Could you check a few things on this model? Use its own coordinates, in mm. A direction names the side the tool comes from. Give positions to 0.01 mm unless a question says otherwise; leave off trailing zeros. Order: outer loops, then holes, each group sorted by start corner. A loop starts at its lowest first (then second) coordinate and runs counter-clockwise, first axis right, second up. Notation, with made-up numbers: (-23, 88) -> (-1, 88) arc R24 ccw to (-1, 113) -> close; hole circle Ø11 at (68.5, 32). An arc over 180 degrees is marked (long way). Write each question's results on one line, items separated by ' | '.
```python
from build123d import *

# Parameters (mm, degrees)
F0_W     = 101.6
F0_H     = 76.2
F1_DEPTH = 76.2
F3_DEPTH = 76.201
F2_W     = 63.5
F2_H     = 25.4
F4_DEPTH = 63.5
F2_W_2   = 12.7
F2_H_2   = 31.75
F5_DEPTH = 50.8
F6_R     = 5.08
F7_R     = 5.08


with BuildPart() as f1:
    # F0 (on Front) → F1 (new body)
    with BuildSketch(Plane.XZ):
        Rectangle(F0_W, F0_H)
    extrude(amount=F1_DEPTH)

    # F2 (on face) → F3 (cut, through all)
    with BuildSketch(Plane.XZ.offset(76.2)):
        with BuildLine():
            ThreePointArc((-25.4, 38.1), (0, 12.7), (25.4, 38.1))
            Line((25.4, 38.1), (-25.4, 38.1))
        make_face()
    extrude(amount=-F3_DEPTH, mode=Mode.SUBTRACT)

    # F2 (on face) → F4 (cut)
    with BuildSketch(Plane.XZ.offset(76.2)):
        with Locations((0, -25.4)):
            Rectangle(F2_W, F2_H)
    extrude(amount=-F4_DEPTH, mode=Mode.SUBTRACT)

    # F2 (on face) → F5 (cut)
    with BuildSketch(Plane.XZ.offset(76.2)):
        Polygon((50.8, 38.1), (27.94, 38.1), (27.94, -6.35), (38.1, -6.35), (50.8, -6.35), align=None)
        with Locations((44.45, -22.225)):
            Rectangle(F2_W_2, F2_H_2)
        Polygon((-27.94, -6.35), (-27.94, 38.1), (-50.8, 38.1), (-50.8, -6.35), (-38.1, -6.35), align=None)
        with Locations((-44.45, -22.225)):
            Rectangle(F2_W_2, F2_H_2)
    extrude(amount=-F5_DEPTH, mode=Mode.SUBTRACT)

    # F6
    f6_edges = [f1.edges().sort_by_distance(p)[0] for p in [
        (27.94, -50.8, -6.35),
        (-27.94, -50.8, -6.35),
    ]]
    fillet(f6_edges, radius=F6_R)

    # F7
    f7_edges = [f1.edges().sort_by_distance(p)[0] for p in [
        (50.8, -12.7, 38.1),
        (-50.8, -12.7, 38.1),
    ]]
    fillet(f7_edges, radius=F7_R)


solid = f1.part
```
Q1. I need wall thicknesses on line 1 along X through (y, z) = (-49.5, -18.5); line 2 along Y through (x, z) = (35, 22); line 3 along Y through (x, z) = (-4, -13). Which ranges of each line are inside material? Lowest first, please.
Here are the results:
line 1: x = -38.1 to -31.75, 31.75 to 38.1 | line 2: y = -25.4 to 0 | line 3: y = -12.7 to 0
Q2. Suppose I cut it at C-C on x = -35. Please give me the cut outline in (y, z).
Here are the results:
outline: (-76.2, -38.1) -> (0, -38.1) -> (0, 38.1) -> (-25.4, 38.1) -> (-25.4, -6.35) -> (-76.2, -6.35) -> close
Q3. For faces 1 (the flat face through (-36, -51, -6.35)), 2 (the flat face through (38.1, -51, -22)), 3 (the flat face through (-31.75, -45, -26)), 4 (the flat face through (36, -51, -6.35)), which set-ups out of +Z, -Z, +X, -X, +Y, -Y let a thin tool reach every point of the face, with its end or its side?
Here are the results:
face 1: +Z, -X, -Y | face 2: +Z, -Z, +X, -Y | face 3: -Z, -Y | face 4: +Z, +X, -Y
Q4. Suppose I cut it at D-D on z = -21.5. Please give me the cut outline in (x, y).
Here are the results:
outline: (-50.8, -25.4) -> (-38.1, -25.4) -> (-38.1, -76.2) -> (-31.75, -76.2) -> (-31.75, -12.7) -> (31.75, -12.7) -> (31.75, -76.2) -> (38.1, -76.2) -> (38.1, -25.4) -> (50.8, -25.4) -> (50.8, 0) -> (-50.8, 0) -> close
Q5. Suppose I cut it at A-A on y = -49. Please give me the cut outline in (x, z), and give its area (3 significant figures).
Here are the results:
outline: (-38.1, -38.1) -> (-31.75, -38.1) -> (-31.75, -12.7) -> (31.75, -12.7) -> (31.75, -38.1) -> (38.1, -38.1) -> (38.1, -6.35) -> (33.02, -6.35) arc R5.08 cw to (27.94, -1.27) -> (27.94, 38.1) -> (25.4, 38.1) arc R25.4 cw to (-25.4, 38.1) -> (-27.94, 38.1) -> (-27.94, -1.27) arc R5.08 cw to (-33.02, -6.35) -> (-38.1, -6.35) -> close | area: 2,290 mm²
Q6. Thinking about a two-plate mould opening in X: for faces 5 (the cylindrical face through (-29.389, -50.444, -4.822)), 6 (the cylindrical face through (49.351, -12.878, 36.572)), 7 (the flat face through (31.75, -45, -26)), which applies, +X half, -X half, draft (parallel to the pull), parting line (faces both ways), or undercut?
Here are the results:
face 5: -X half | face 6: +X half | face 7: undercut
Q7. I'm going to push flat-ended pins straight in: pin 1 Ø12 at (y, z) = (-61, 16.5) entering from +X; pin 2 Ø2 at (x, y) = (0.5, -12) entering from +Z; pin 3 Ø7 at (x, z) = (-34, 3) entering from -Y; pin 4 Ø12 at (x, z) = (12.5, 29.5) entering from -Y. Where does each tip first touch, or does it pass through?
Here are the results:
pin 1: stops at x = 27.94 | pin 2: stops at z = 12.74 | pin 3: stops at y = -25.4 | pin 4: passes through
Q8. Suppose I cut it at B-B on z = -10. Please give me the cut outline in (x, y), and give its area (3 significant figures).
Here are the results:
outline: (-50.8, -25.4) -> (-38.1, -25.4) -> (-38.1, -76.2) -> (38.1, -76.2) -> (38.1, -25.4) -> (50.8, -25.4) -> (50.8, 0) -> (-50.8, 0) -> close | area: 6,450 mm²
